Geometry: final body of the model. Coordinates: model frame, mm. A direction names the side the tool comes from. Give positions to 0.01 mm unless a question says otherwise; leave off trailing zeros. Order: outer loops, then holes, each group sorted by start corner. A loop starts at its lowest first (then second) coordinate and runs counter-clockwise, first axis right, second up. Notation, with made-up numbers: (-40, -37.75) - (18, -37.75) arc R26 ccw to (18, -5.75) - close; hole circle Ø9 at (-33, -5). An arc over 180 degrees is marked (long way). Put each result on its own line as item: value. Start each with the question number.
1. Section C-C on x = 27.35. Return the cut outline in (y, z).
2. Section B-B on z = 2. Return the cut outline in (x, y), plus the area to 3 significant figures.
3. Set-up query: faces 5 (the flat face through (51.724, 102, 6)), 6 (the flat face through (54.234, 102, 6)), 7 (the flat face through (2.8, 38, 2)), 8 (the cylindrical face through (29.4, 13.47, 0.94)). Return all of +Z, -Z, +X, -X, +Y, -Y with unobstructed straight access to the full face (end or side cutting, diameter ignored); none if empty.
4. Section D-D on y = 108. Return the cut outline in (x, z).
5. Mould query, pull axis Y, two halves, no side actions, for faces 1 (the flat face through (1, 77.3, 6)), 2 (the flat face through (2.51, 102, 6)), 3 (the cylindrical face through (27.07, 66.356, 0.944)), 4 (the flat face through (27, 127, -2)). Classes: pulls with the +Y half, pulls with the -Y half, needs draft (parallel to the pull), parting line crosses it, or undercut.
6. Section A-A on z = 10.5. Return the cut outline in (x, y).
7. First-contact query: P1, Ø22.5, axis at x = 25, y = 30.5, coming from the +Z side; P2, Ø10, axis at y = 80.5, z = 9, coming from the +X side; P3, Ø1.5, axis at y = 21.5, z = 3.5, coming from the -X side; P4, Ø2, axis at x = 42, z = 7, coming from the -Y side. Flat tips, straight axial feed; report the tip coordinate or a pass-through.
8. Ray query, line 1 along Y through (x, z) = (27.35, -1); line 2 along Y through (x, z) = (27.35, 3); line 3 along X through (y, z) = (13, 2.25). Return the intervals inside material, ascending. Write a range as from..to.
from build123d import *

# Parameters (mm, degrees)
SKETCH_W      = 54.7
SKETCH_H      = 127
PAD_DEPTH     = 5
SKETCH001_W   = 49.1
SKETCH001_H   = 71.4
SKETCH001_R   = 2.15
SKETCH001_R_2 = 22.5
PAD001_DEPTH  = 5
SKETCH002_R   = 2.15
SKETCH002_R_2 = 22.5
POCKET_DEPTH  = 3
SKETCH003_W   = 2.51
SKETCH003_H   = 49.7
PAD002_DEPTH  = 12


with BuildPart() as part:
    # Sketch → Pad (new body)
    with BuildSketch(Plane.XY):
        with Locations((27.35, 63.5)):
            Rectangle(SKETCH_W, SKETCH_H)
    extrude(amount=-PAD_DEPTH)

    # Sketch001 → Pad001 (join)
    with BuildSketch(Plane.XY):
        with Locations((27.35, 38.5)):
            Rectangle(SKETCH001_W, SKETCH001_H)
        with Locations((27.35, 12.823933)):
            Circle(SKETCH001_R, mode=Mode.SUBTRACT)
        with Locations((27.35, 64.223933)):
            Circle(SKETCH001_R, mode=Mode.SUBTRACT)
        with Locations((27.35, 38.523933)):
            Circle(SKETCH001_R_2, mode=Mode.SUBTRACT)
    extrude(amount=PAD001_DEPTH)

    # Sketch002 → Pocket (cut)
    with BuildSketch(Plane.XY):
        with Locations((27.35, 12.823933)):
            Circle(SKETCH002_R)
        with Locations((27.35, 64.223933)):
            Circle(SKETCH002_R)
        with Locations((27.35, 38.523933)):
            Circle(SKETCH002_R_2)
    extrude(amount=-POCKET_DEPTH, mode=Mode.SUBTRACT)

    # Sketch003 → Pad002 (join)
    with BuildSketch(Plane.XY):
        with Locations((1.255, 102.15)):
            Rectangle(SKETCH003_W, SKETCH003_H)
        with Locations((52.979469, 102.15)):
            Rectangle(SKETCH003_W, SKETCH003_H)
    extrude(amount=PAD002_DEPTH)


solid = part.part
Resolved:
1. outline: (0, -5) - (127, -5) - (127, 0) - (74.2, 0) - (74.2, 5) - (66.37, 5) - (66.37, -3) - (62.07, -3) - (62.07, 5) - (61.02, 5) - (61.02, -3) - (16.02, -3) - (16.02, 5) - (14.97, 5) - (14.97, -3) - (10.67, -3) - (10.67, 5) - (2.8, 5) - (2.8, 0) - (0, 0) - close
2. outline: (0, 77.3) - (2.51, 77.3) - (2.51, 127) - (0, 127) - close; (2.8, 2.8) - (51.9, 2.8) - (51.9, 74.2) - (2.8, 74.2) - close; (51.72, 77.3) - (54.23, 77.3) - (54.23, 127) - (51.72, 127) - close; hole circle Ø45 at (27.35, 38.52); hole circle Ø4.3 at (27.35, 12.82); hole circle Ø4.3 at (27.35, 64.22)
2. area: 2,140 mm^2
3. face 5: +Z, +Y
3. face 6: +Z, +X, +Y, -Y
3. face 7: +Z, -X, +Y, -Y
3. face 8: +Z
4. outline: (0, -5) - (54.7, -5) - (54.7, 0) - (54.23, 0) - (54.23, 12) - (51.72, 12) - (51.72, 0) - (2.51, 0) - (2.51, 12) - (0, 12) - close
5. face 1: pulls with the -Y half
5. face 2: needs draft
5. face 3: undercut
5. face 4: pulls with the +Y half
6. outline: (0, 77.3) - (2.51, 77.3) - (2.51, 127) - (0, 127) - close; (51.72, 77.3) - (54.23, 77.3) - (54.23, 127) - (51.72, 127) - close
7. P1: z = -3
7. P2: x = 54.23
7. P3: x = 2.8
7. P4: through
8. line 1: 0..10.67, 14.97..16.02, 61.02..62.07, 66.37..127
8. line 2: 2.8..10.67, 14.97..16.02, 61.02..62.07, 66.37..74.2
8. line 3: 2.8..25.21, 29.49..51.9
